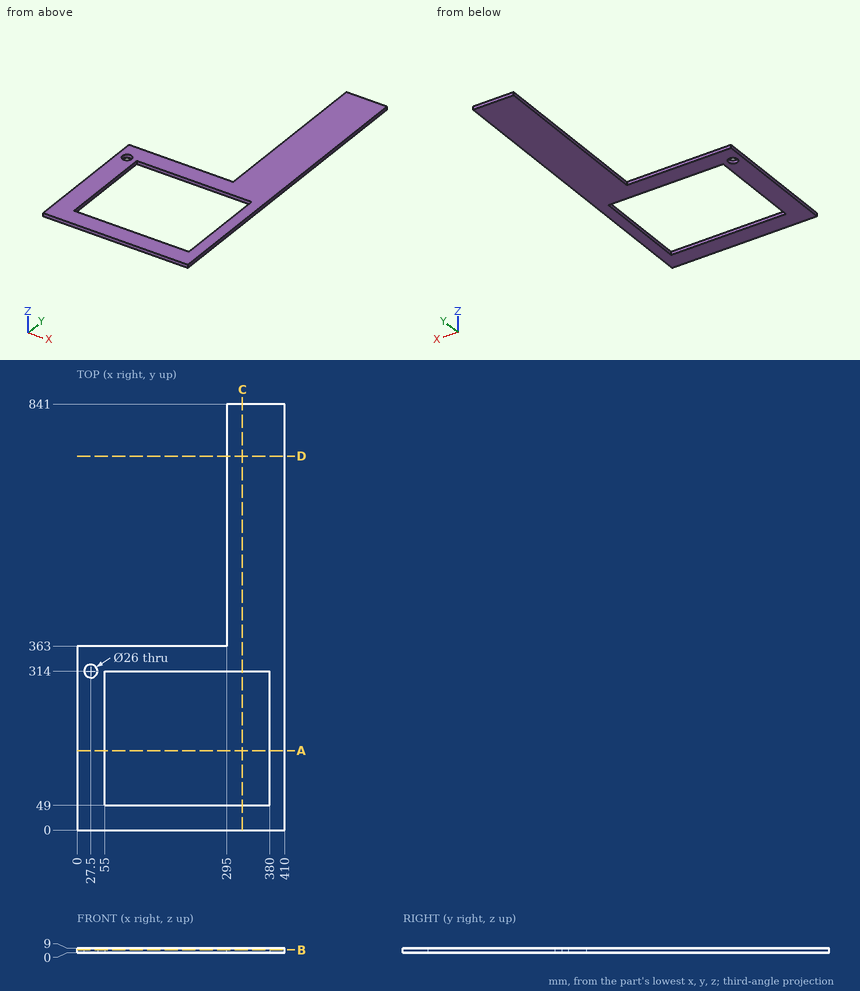
Source: three-view drawing plus pictorial views. Frame: mm from the lowest corner of the part. Give positions to 0.01 mm unless a question says otherwise; leave off trailing zeros. Order: outer loops, then holes, each group sorted by start corner. A loop starts at its lowest first (then second) coordinate and runs counter-clockwise, first axis right, second up. Notation, with made-up numbers: M -11.5,59 L -3.5,59 A15 ccw -3.5,75 Z; hole C -36.5,88 d3. An arc over 180 degrees is marked long. Return JSON: item names as keys, results as strings.
Item 1: Cut plane D-D (y = 738). Return loops of the section in (x, z), then the cut area to 4 significant figures.
Solutions:
{"outline": "M 295,0 L 410,0 L 410,9 L 295,9 Z", "area": "1,035 mm^2"}
Item 2: Cut plane C-C (x = 326.5). Return loops of the section in (y, z).
Solutions:
{"outline": "M 0,0 L 49,0 L 49,9 L 0,9 Z; M 314,0 L 841,0 L 841,9 L 314,9 Z"}
Item 3: Cut plane A-A (y = 157). Return loops of the section in (x, z).
Solutions:
{"outline": "M 0,0 L 55,0 L 55,9 L 0,9 Z; M 380,0 L 410,0 L 410,9 L 380,9 Z"}
Item 4: First-contact query: P1, Ø2, axis at y = 506.5, z = 4.5, coming from the -X side; P2, Ø4.5, axis at x = 197, z = 5.5, coming from the +Y side. Flat tips, straight axial feed; report the tip coordinate or a pass-through.
Solutions:
{"P1": "x = 295", "P2": "y = 363"}
Item 5: Cut plane B-B (z = 5.5). Return loops of the section in (x, y), then the cut area to 3 significant figures.
Solutions:
{"outline": "M 0,0 L 410,0 L 410,841 L 295,841 L 295,363 L 0,363 Z; hole C 27.5,314 d26; hole M 55,49 L 380,49 L 380,314 L 55,314 Z", "area": "117,000 mm^2"}
Item 6: Ray query, probe 1 along Y at (x, z) = (243, 3.75); probe 2 along X at (y, z) = (58, 3.75); probe 3 along X at (y, z) = (311, 5). Return the intervals inside material, ascending.
Solutions:
{"probe 1": "0 to 49, 314 to 363", "probe 2": "0 to 55, 380 to 410", "probe 3": "0 to 14.85, 40.15 to 55, 380 to 410"}
